Work out the finished part from the listing and answer in its coordinate system (mm). Face numbers are marked on the shaded views. A direction names the side the tool comes from. Coordinates: 2 decimals unless noted, no trailing zeros. Loops run counter-clockwise (first coordinate to the right, second up) from the corner with the lowest first, then second, coordinate; pieces in that order, holes last. Notation, with made-up numbers: (39.25, 62.5) - (56.25, 62.5) arc R11 ccw to (56.25, 82.5) - close; hole circle Ø9 at (68, 40.25). An arc over 180 degrees is marked (long way). Write each question's results on one line, items separated by ' | '. Start each with the question number.
Item 1: Section D-D, the plane z = 2.5 is taken. Write down the section's boundary in (x, y).
Item 2: Section A-A, the plane x = 0.4 is taken. Write down the section's boundary in (y, z), plus the area to 3 significant figures.
Item 3: A tool of negligible diameter and unlimited length cuts with its end or side. For the marked faces 1, 2 and 3, from which of +Z, -Z, +X, -X, +Y, -Y can it reach the whole face along a straight path? Write none if from no direction.
Item 4: For a pull along Y with two mould halves and no side action, classify the marked faces 4 and 5 as +Y half, -Y half, draft (parallel to the pull), parting line (faces both ways), or undercut.
Item 5: Each of these flat-tipped pins is pushed along its axis until it touches: pin 1 Ø2 at (y, z) = (14, 0) entering from -X; pin 2 Ø1 at (x, y) = (-0.5, -0.5) entering from -Z. Where does it stop, or does it pass through?
Item 6: Section C-C, the plane z = -1 is taken. Write down the section's boundary in (x, y).
Item 7: Section B-B, the plane y = 14 is taken. Write down the section's boundary in (x, z).
Item 8: Consider probe 1 along Y at (x, z) = (0, 0); probe 2 along Z at (x, y) = (-0.1, -14); probe 3 along Z at (x, y) = (-0.5, 4.5). Determine where each line is inside the solid, lowest interval first. Write a range as [from, to].
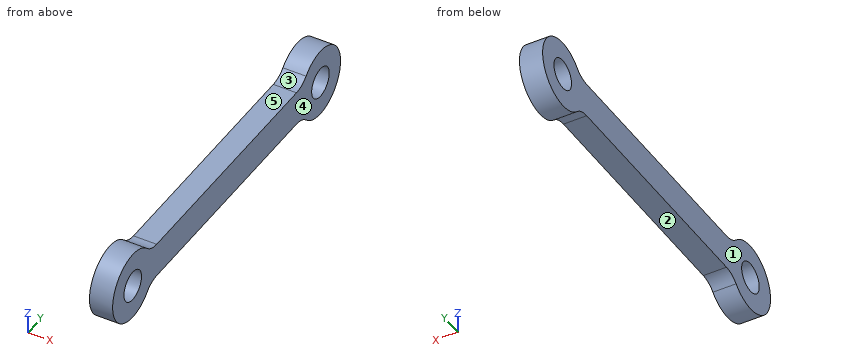
Autodesk Inventor part; units mm, degrees
ref_plane "YZ Plane" through (0, 0, 0) normal (1, 0, 0) x (0, 1, 0)
ref_plane "XZ Plane" through (0, 0, 0) normal (0, 1, 0) x (-1, 0, 0)
ref_plane "XY Plane" through (0, 0, 0) normal (0, 0, 1) x (1, 0, 0)
sketch "Sketch1" plane through (0, 0, 0) normal (1, 0, 0) x (0, 1, 0)
  line L0 (-14, 0) -> (14, 0) construction
  circle A0 centre (-14, 0) radius 3
  circle A1 centre (14, 0) radius 3
  line L1 (-11.4019, 1.5) -> (11.4019, 1.5)
  line L2 (11.4019, -1.5) -> (-11.4019, -1.5)
  point P0 (0, 0)
  point P1 (0, 0)
  dimension "d0" = 28
  dimension "d1" = 6
  dimension "d2" = 3
extrude "Extrusion1" add sketch "Sketch1" along normal mid plane 2
fillet "Fillet1" radius 2 4 edges at (0, -11.4019, 1.5) (0, -11.4019, -1.5) (0, 11.4019, -1.5) (0, 11.4019, 1.5)
sketch "Sketch2" plane through (1, 0, 0) normal (1, 0, 0) x (0, 0, -1)
  arc A0 (-2.1, -11.8576) -> (2.1, -11.8576) centre (0, -14) ccw
  arc A1 (1.5, -10.4293) -> (2.1, -11.8576) centre (3.5, -10.4293) ccw
  line L0 (1.5, -10.4293) -> (1.5, 10.4293)
  arc A2 (2.1, 11.8576) -> (1.5, 10.4293) centre (3.5, 10.4293) ccw
  arc A3 (2.1, 11.8576) -> (-2.1, 11.8576) centre (0, 14) ccw
  arc A4 (-1.5, 10.4293) -> (-2.1, 11.8576) centre (-3.5, 10.4293) ccw
  line L1 (-1.5, 10.4293) -> (-1.5, -10.4293)
  arc A5 (-2.1, -11.8576) -> (-1.5, -10.4293) centre (-3.5, -10.4293) ccw
  point P0 (0, 0)
hole "Hole1" at (1, -14, 0) at (1, 14, 0) direction (-1, 0, 0) diameter 2.621 end through all
properties part number "Backplane_Nut" material "Aluminum 6061"
Answer key:
1) outline: (-1, -15.66) - (1, -15.66) - (1, -12.34) - (-1, -12.34) - close; (-1, 12.34) - (1, 12.34) - (1, 15.66) - (-1, 15.66) - close
2) outline: (-11.86, -2.1) arc R2 cw to (-10.43, -1.5) - (10.43, -1.5) arc R2 cw to (11.86, -2.1) arc R3 ccw (long way) to (11.86, 2.1) arc R2 cw to (10.43, 1.5) - (-10.43, 1.5) arc R2 cw to (-11.86, 2.1) arc R3 ccw (long way) to start; hole circle Ø2.62 at (-14, 0); hole circle Ø2.62 at (14, 0) | area: 113 mm^2
3) face 1: +Z, -Z, -X, +Y, -Y | face 2: -Z, +X, -X | face 3: +Z, +X, -X
4) face 4: draft | face 5: undercut
5) pin 1: passes through | pin 2: stops at z = -1.5
6) outline: (-1, -16.83) - (1, -16.83) - (1, -14.85) - (-1, -14.85) - close; (-1, -13.15) - (1, -13.15) - (1, 13.15) - (-1, 13.15) - close; (-1, 14.85) - (1, 14.85) - (1, 16.83) - (-1, 16.83) - close
7) outline: (-1, -3) - (1, -3) - (1, -1.31) - (-1, -1.31) - close; (-1, 1.31) - (1, 1.31) - (1, 3) - (-1, 3) - close
8) probe 1: y = [-17, -15.31], [-12.69, 12.69], [15.31, 17] | probe 2: z = [-3, -1.31], [1.31, 3] | probe 3: z = [-1.5, 1.5]
